```python
from build123d import *

# Parameters (mm, degrees)
SKETCH1_R           = 8
BOSS_EXTRUDE1_DEPTH = 4
SKETCH2_W           = 40
SKETCH2_H           = 10
BOSS_EXTRUDE2_DEPTH = 32
SKETCH3_R           = 15
SKETCH3_R_2         = 10
BOSS_EXTRUDE3_DEPTH = 10
BOSS_EXTRUDE4_DEPTH = 10
RIB6_REACH          = 99.35
SKETCH5_WALL_W      = 246.096125016
SKETCH5_WALL_H      = 10


with BuildPart() as part:
    # Sketch1 → Boss-Extrude1 (new, symmetric)
    with BuildSketch(Plane(origin=(0, 0, 0), x_dir=(1, 0, 0), z_dir=(0, 1, 0))):
        with BuildLine():
            Line((-28, 18), (28, 18))
            ThreePointArc((28, 18), (46, 0), (28, -18))
            Line((28, -18), (-28, -18))
            ThreePointArc((-28, -18), (-46, 0), (-28, 18))
        make_face()
        with Locations(Location((-28, 0, 0), (0, 0, 270))):
            Circle(SKETCH1_R, mode=Mode.SUBTRACT)
        with Locations(Location((28, 0, 0), (0, 0, 270))):
            Circle(SKETCH1_R, mode=Mode.SUBTRACT)
    extrude(amount=BOSS_EXTRUDE1_DEPTH, both=True)

    # Sketch2 → Boss-Extrude2 (add)
    with BuildSketch(Plane(origin=(0, 4, 0), x_dir=(1, 0, 0), z_dir=(0, 1, 0))):
        with Locations((0, 13)):
            Rectangle(SKETCH2_W, SKETCH2_H)
    extrude(amount=BOSS_EXTRUDE2_DEPTH)



with BuildPart() as body_2:
    # Sketch3 → Boss-Extrude3 (new, symmetric)
    with BuildSketch(Plane(origin=(0, 46, 0), x_dir=(1, 0, 0), z_dir=(0, 1, 0))):
        with Locations(Location((0, 50, 0), (0, 0, 270))):
            Circle(SKETCH3_R)
        with Locations(Location((0, 50, 0), (0, 0, 270))):
            Circle(SKETCH3_R_2, mode=Mode.SUBTRACT)
    extrude(amount=BOSS_EXTRUDE3_DEPTH, both=True)


with BuildPart() as part_1:
    add(part.part)

    add(body_2.part)  # Boss-Extrude4 merges body 2
    # Sketch4 → Boss-Extrude4 (add)
    with BuildSketch(Plane(origin=(0, 46, 0), x_dir=(1, 0, 0), z_dir=(0, 1, 0))):
        with BuildLine():
            Line((20, 8), (20, 18))
            Line((20, 18), (14.831993052, 52.238745657))
            ThreePointArc((14.831993052, 52.238745657), (0, 35), (-14.831993052, 52.238745657))
            Line((-14.831993052, 52.238745657), (-20, 18))
            Line((-20, 18), (-20, 8))
            Line((-20, 8), (20, 8))
        make_face()
    extrude(amount=-BOSS_EXTRUDE4_DEPTH)

    # Sketch5 wall → Rib6 (add, up to next)
    with BuildSketch(Plane(origin=(0, 25, 5), x_dir=(0, -0.850265146688, 0.526354614616), z_dir=(0, -0.526354614616, -0.850265146688)), mode=Mode.PRIVATE) as rib6_sk1:
        Rectangle(SKETCH5_WALL_W, SKETCH5_WALL_H)
    rib6_tool1 = extrude(rib6_sk1.sketch, amount=RIB6_REACH, mode=Mode.PRIVATE) - part_1.part
    add(rib6_tool1.solids().sort_by_distance((0, 25, 5))[0])


solid = part_1.part
```
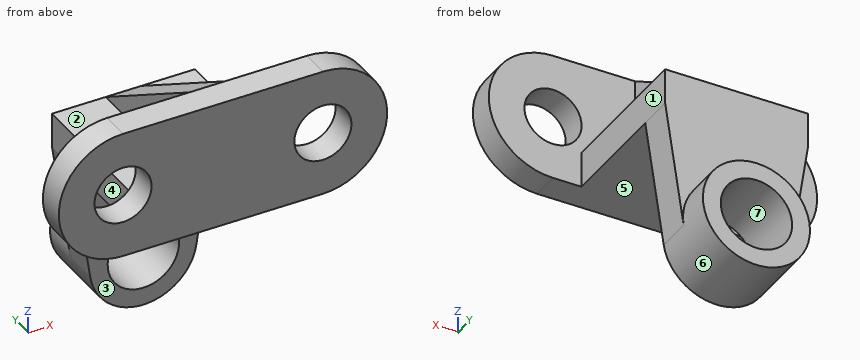
Geometry check sheet. Reference: the model listing, model coordinates, mm. Face numbers are marked on the shaded views. A direction names the side the tool comes from. Coordinates: 2 decimals unless noted, no trailing zeros. Write each loop counter-clockwise with the first axis right and the second up, starting at its lowest first coordinate (ties: lowest second). Pieces come first, ordered by that corner, then holes. Notation, with made-up numbers: M -14,77.25 L 35,77.25 A28 cw 35,98.25 Z; hole C -30.5,25 d10. An arc over 180 degrees is marked long. One line per item, written item: value. Start each with the question number.
(1) Sectioned sample at D-D, the plane z = -5. Enter the section's corners in (x, y) (3 decimals), and give its area (3 significant figures).
(2) Sectioned sample at A-A, the plane x = 0. Enter the section's corners in (y, z).
(3) Tool access check on the marked faces 1, 2, 3 and 4. Record the directions out of +Z, -Z, +X, -X, +Y, -Y that give a thin tool (end or side, any length) a straight path to the whole face; none if there is none.
(4) Sectioned sample at C-C, the plane y = 31. Enter the section's corners in (x, z), and give its area (3 significant figures).
(5) Depth check by flat-ended pin: pin 1 (5 mm diameter, centred on y = 26.5, z = -15.5, fed in from -X); pin 2 (7.5 mm diameter, centred on x = 13, y = 19, fed in from +Z); pin 3 (11 mm diameter, centred on y = 21.5, z = -15, fed in from +X); pin 4 (21 mm diameter, centred on x = 28, z = 0, fed in from -Y). Enter the tip coordinate at first touch or a pass-through.
(6) Scan lines: line 1 along X through (y, z) = (0, 0); line 2 along Y through (x, z) = (2, -38.5); line 3 along Y through (x, z) = (-28, 9). Record each from-to range of solid material in increasing order. Write a range as [from, to].
(7) Sectioned sample at B-B, the plane z = -49.5. Enter the section's corners in (x, y), and give its area (3 significant figures).
(8) Release check for a two-part mould opening along X. For the marked faces 5, 6 and 7 record: released by +X, released by -X, zero draft, split by the parting line, or undercut.
Filled sheet:
1. outline: M -45.292,-4 L -34.245,-4 L -34.245,4 L -45.292,4 Z; M -21.755,-4 L 21.755,-4 L 21.755,4 L 5,4 L 5,41.154 L -5,41.154 L -5,4 L -21.755,4 Z; M 34.245,-4 L 45.292,-4 L 45.292,4 L 34.245,4 Z
1. area: 896 mm²
2. outline: M -4,-18 L 36,-18 L 36,-40 L 56,-40 L 56,-35 L 46,-35 L 46,-8 L 4,18 L -4,18 Z; M 36,-65 L 56,-65 L 56,-60 L 36,-60 Z
3. face 1: +Z, -Z, +X, +Y
3. face 2: +Z, -X, +Y
3. face 3: -Z, +X, -X, -Y
3. face 4: +Z, -Z, -X, +Y
4. outline: M -20,-18 L 20,-18 L 20,-8 L 5,-8 L 5,1.29 L -5,1.29 L -5,-8 L -20,-8 Z
4. area: 493 mm²
5. pin 1: x = -20
5. pin 2: z = -8
5. pin 3: x = 20
5. pin 4: y = -4
6. line 1: [-46, -36], [-20, 20], [36, 46]
6. line 2: [36, 56]
6. line 3: [-4, 4]
7. outline: M -15.25,36 L -9.99,36 L -9.99,56 L -14.99,56 L -14.99,46 L -15.25,46 Z; M 9.99,36 L 15.25,36 L 15.25,46 L 14.99,46 L 14.99,56 L 9.99,56 Z
7. area: 205 mm²
8. face 5: zero draft
8. face 6: split by the parting line
8. face 7: undercut
